Check sheet for the modelled part. Datum: model origin and axes. Units: mm. A direction names the side the tool comes from. Round coordinates to 2 decimals unless told otherwise and drop trailing zeros. Order: outer loops, then holes, each group sorted by start corner. A loop starts at its lowest first (then second) coordinate and runs counter-clockwise, first axis right, second up. Notation, with made-up numbers: (-34, 88.25) -> (25, 88.25) arc R14 cw to (25, 103.25) -> close; hole circle Ø9 at (35.25, 20.5). An arc over 180 degrees is marked (long way). Answer in a Markdown table with one row per item.
```python
from build123d import *

# Parameters (mm, degrees)
F1_R     = 9
F2_DEPTH = 3
F0_R     = 2
F3_DEPTH = 5
F4_DEPTH = 5


with BuildPart() as f2:
    # F1 (on Top) → F2 (new body)
    with BuildSketch(Plane.XY):
        with BuildLine():
            ThreePointArc((76.4386732788, -130.3071677685), (85.4189293999, -126.5874238895), (89.1386732788, -117.6071677685))
            Line((89.1386732788, -117.6071677685), (89.1386732788, 176.8828322315))
            ThreePointArc((89.1386732788, 176.8828322315), (85.4189293999, 185.8630883526), (76.4386732788, 189.5828322315))
            Line((76.4386732788, 189.5828322315), (-77.3583267212, 189.5828322315))
            ThreePointArc((-77.3583267212, 189.5828322315), (-86.3385828423, 185.8630883526), (-90.0583267212, 176.8828322315))
            Line((-90.0583267212, 176.8828322315), (-90.0583267212, -117.6071677685))
            ThreePointArc((-90.0583267212, -117.6071677685), (-86.3385828423, -126.5874238895), (-77.3583267212, -130.3071677685))
            Line((-77.3583267212, -130.3071677685), (76.4386732788, -130.3071677685))
        make_face()
        with Locations((-67.1983267212, -97.2871677685)):
            Circle(F1_R, mode=Mode.SUBTRACT)
        with Locations((66.2786732788, -97.2871677685)):
            Circle(F1_R, mode=Mode.SUBTRACT)
        with Locations((-67.1983267212, 156.5628322315)):
            Circle(F1_R, mode=Mode.SUBTRACT)
        with Locations((66.2786732788, 156.5628322315)):
            Circle(F1_R, mode=Mode.SUBTRACT)
    extrude(amount=F2_DEPTH)

    # F0 (on Top) → F3 (join)
    with BuildSketch(Plane.XY):
        with BuildLine():
            add(Edge.make_bspline(
                [(44.5225109401, 51.6328074749), (31.7931699117, 61.9046377655), (15.5430863667, 67.5611001635), (-0.8466675809, 67.3154957518)],
                knots=[0, 0, 0, 0, 1, 1, 1, 1], degree=3))
            add(Edge.make_bspline(
                [(-0.8466675809, 67.3154957518), (-16.6914552758, 67.2139309121), (-32.3557233009, 61.5656679848), (-44.6624829203, 51.6328074749)],
                knots=[0, 0, 0, 0, 1, 1, 1, 1], degree=3))
            Line((-44.6624829203, 51.6328074749), (-31.2156959628, 36.0207258387))
            add(Edge.make_bspline(
                [(-31.2156959628, 36.0207258387), (-19.8668770846, 44.9768453315), (-4.5754724959, 48.626535939), (9.607211652, 45.8069907111)],
                knots=[0, 0, 0, 0, 1, 1, 1, 1], degree=3))
            add(Edge.make_bspline(
                [(9.607211652, 45.8069907111), (17.4015278884, 44.3075346269), (24.8181773865, 40.8851063357), (31.0757239826, 36.0207258387)],
                knots=[0, 0, 0, 0, 1, 1, 1, 1], degree=3))
            Line((31.0757239826, 36.0207258387), (44.5225109401, 51.6328074749))
        make_face()
        with Locations((-31.2156959628, 48.4397840007)):
            Circle(F0_R, mode=Mode.SUBTRACT)
        with Locations((31.0757239826, 48.4397840007)):
            Circle(F0_R, mode=Mode.SUBTRACT)
    extrude(amount=F3_DEPTH)

    # F0 (on Top) → F4 (join)
    with BuildSketch(Plane.XY):
        with BuildLine():
            add(Edge.make_bspline(
                [(-48.3654487285, 48.4397840007), (-48.5903470483, 48.2253463108), (-48.8152456845, 48.0109111522), (-49.0401417893, 47.7964712472)],
                knots=[0, 0, 0, 0, 1, 1, 1, 1], degree=3))
            add(Edge.make_bspline(
                [(-49.0401417893, 47.7964712472), (-63.2089023734, 34.4854490825), (-71.5164935114, 15.1358143832), (-71.2536124009, -4.3823817258)],
                knots=[0, 0, 0, 0, 1, 1, 1, 1], degree=3))
            add(Edge.make_bspline(
                [(-71.2536124009, -4.3823817258), (-71.2452113687, -24.6424367519), (-62.0032950914, -44.5436607549), (-46.6551817954, -57.7066801488)],
                knots=[0, 0, 0, 0, 1, 1, 1, 1], degree=3))
            add(Edge.make_bspline(
                [(-46.6551817954, -57.7066801488), (-32.4680977849, -70.1146960954), (-13.1730887798, -76.4354807885), (5.6641111211, -74.8365011098)],
                knots=[0, 0, 0, 0, 1, 1, 1, 1], degree=3))
            add(Edge.make_bspline(
                [(5.6641111211, -74.8365011098), (26.0758546138, -73.3164411383), (45.4498377508, -62.4142271403), (57.4270848419, -45.8498931001)],
                knots=[0, 0, 0, 0, 1, 1, 1, 1], degree=3))
            add(Edge.make_bspline(
                [(57.4270848419, -45.8498931001), (69.0851876389, -30.1089858288), (73.6526652184, -9.3511818312), (69.782774857, 9.8980318978)],
                knots=[0, 0, 0, 0, 1, 1, 1, 1], degree=3))
            add(Edge.make_bspline(
                [(69.782774857, 9.8980318978), (66.9379075577, 24.63337834), (59.2125294632, 38.289509842), (48.2254770647, 48.4397840007)],
                knots=[0, 0, 0, 0, 1, 1, 1, 1], degree=3))
            Line((48.2254770647, 48.4397840007), (34.7786901072, 32.8277023646))
            add(Edge.make_bspline(
                [(34.7786901072, 32.8277023646), (45.6135961749, 22.6148903531), (51.529750139, 7.5398526857), (50.4143066574, -7.3322188933)],
                knots=[0, 0, 0, 0, 1, 1, 1, 1], degree=3))
            add(Edge.make_bspline(
                [(50.4143066574, -7.3322188933), (49.9263728127, -14.7005793852), (47.7863498942, -21.9724011014), (44.1694752054, -28.4438325965)],
                knots=[0, 0, 0, 0, 1, 1, 1, 1], degree=3))
            Line((44.1694752054, -28.4438325965), (16.765956425, -1.9739032718))
            Line((16.765956425, -1.9739032718), (2.9398510008, 27.8290335048))
            Line((2.9398510008, 27.8290335048), (2.919062006, -17.3035535989))
            Line((2.919062006, -17.3035535989), (30.6128555902, -44.1029862757))
            add(Edge.make_bspline(
                [(30.6128555902, -44.1029862757), (18.2719055103, -53.691098487), (1.3390673943, -56.8712473399), (-13.6652661742, -52.6212601112)],
                knots=[0, 0, 0, 0, 1, 1, 1, 1], degree=3))
            add(Edge.make_bspline(
                [(-13.6652661742, -52.6212601112), (-19.7747362729, -50.9170276822), (-25.5600477213, -48.0575679008), (-30.5880749451, -44.220664643)],
                knots=[0, 0, 0, 0, 1, 1, 1, 1], degree=3))
            Line((-30.5880749451, -44.220664643), (-2.7059963529, -17.3035535989))
            add(Edge.make_bspline(
                [(-2.7059963529, -17.3035535989), (-2.7546011493, -2.6300403353), (-2.535721196, 13.2099469053), (-2.7061599436, 27.8775294516)],
                knots=[0, 0, 0, 0, 1, 1, 1, 1], degree=3))
            Line((-2.7061599436, 27.8775294516), (-16.5528929868, -1.9739029554))
            Line((-16.5528929868, -1.9739029554), (-44.1917691347, -28.6635004431))
            add(Edge.make_bspline(
                [(-44.1917691347, -28.6635004431), (-52.6237632628, -13.9439238932), (-52.8254617605, 5.0855102919), (-44.7095549634, 19.9693104078)],
                knots=[0, 0, 0, 0, 1, 1, 1, 1], degree=3))
            add(Edge.make_bspline(
                [(-44.7095549634, 19.9693104078), (-42.1723888347, 24.7374657043), (-38.8143418771, 29.0889415146), (-34.9186624038, 32.8277023646)],
                knots=[0, 0, 0, 0, 1, 1, 1, 1], degree=3))
            Line((-34.9186624038, 32.8277023646), (-48.3654487285, 48.4397840007))
        make_face()
        with Locations((0.0002132058, -64.9058073759)):
            Circle(F0_R, mode=Mode.SUBTRACT)
        with Locations((-60.7696250081, 0)):
            Circle(F0_R, mode=Mode.SUBTRACT)
        with Locations((61.1233077943, 0)):
            Circle(F0_R, mode=Mode.SUBTRACT)
    extrude(amount=F4_DEPTH)


solid = f2.part
```
(1) Scan lines: probe 1 along X at (y, z) = (0, 3.55); probe 2 along Y at (x, z) = (-14.5, 4.5); probe 3 along Y at (x, z) = (-22, 3.6). Record each from-to range of solid material in increasing order. Write a range as from..to.
Solutions:
| item | result |
|---|---|
| probe 1 | -71.17..-62.77, -58.77..-50.52, -15.64..-2.68, 2.93..15.85, 50.4..59.12, 63.12..71.03 |
| probe 2 | -73.59..-52.38, -28.69..2.45, 44.63..65.86 |
| probe 3 | -71.6..-49.48, -35.93..-7.23, 41.75..63.87 |
(2) Depth check by flat-ended pin: pin 1 Ø2 at (x, y) = (60.5, -0.5) entering from +Z. Enter the tip coordinate at first touch or a pass-through.
Solutions:
| item | result |
|---|---|
| pin 1 | z = 3 |
(3) Draft check along Y on faces 3 (the flat face through (-16.84, -30.95, 3.99)), 4 (the flat face through (16, -27, 5)), 5 (the cylindrical face through (85.32, -126.686, 1.479)), 6 (the flat face through (-9.533, 13.161, 3.986)). Enter one of: pulls with the +Y half, pulls with the -Y half, needs draft (parallel to the pull), parting line crosses it, or undercut.
Solutions:
| item | result |
|---|---|
| face 3 | undercut |
| face 4 | needs draft |
| face 5 | pulls with the -Y half |
| face 6 | undercut |
(4) Section check B-B on z = 2.2. Record the boundary of the cut face in (x, y).
Solutions:
| item | result |
|---|---|
| outline | (-90.06, -117.61) arc R12.7 ccw to (-77.36, -130.31) -> (76.44, -130.31) arc R12.7 ccw to (89.14, -117.61) -> (89.14, 176.88) arc R12.7 ccw to (76.44, 189.58) -> (-77.36, 189.58) arc R12.7 ccw to (-90.06, 176.88) -> close; hole circle Ø18 at (-67.2, -97.29); hole circle Ø18 at (-67.2, 156.56); hole circle Ø18 at (66.28, -97.29); hole circle Ø18 at (66.28, 156.56) |
(5) Tool access check on faces 1 (the flat face through (41.596, 40.743, 3.986)), 2 (the cylindrical face through (-63, 148.6, 1.5)). Record the directions out of +Z, -Z, +X, -X, +Y, -Y that give a thin tool (end or side, any length) a straight path to the whole face; none if there is none.
Solutions:
| item | result |
|---|---|
| face 1 | +Z |
| face 2 | +Z, -Z |
(6) Section check C-C on y = -82. Record the boundary of the cut face in (x, z).
Solutions:
| item | result |
|---|---|
| outline | (-90.06, 0) -> (89.14, 0) -> (89.14, 3) -> (-90.06, 3) -> close |
(7) Section check A-A on y = 160. Record the boundary of the cut face in (x, z), plus the area to 3 significant figures.
Solutions:
| item | result |
|---|---|
| outline | (-90.06, 0) -> (-75.52, 0) -> (-75.52, 3) -> (-90.06, 3) -> close; (-58.88, 0) -> (57.96, 0) -> (57.96, 3) -> (-58.88, 3) -> close; (74.6, 0) -> (89.14, 0) -> (89.14, 3) -> (74.6, 3) -> close |
| area | 438 mm^2 |
